from build123d import *

# Parameters (mm, degrees)
BOSS_EXTRUDE1_DEPTH     = 10
CUT_EXTRUDE1_DEPTH      = 44.76694614
CUT_EXTRUDE1_DEPTH_BACK = 44.76694614
SKETCH2_R               = 2.5


with BuildPart() as part:
    # Sketch1 → Boss-Extrude1 (new body)
    with BuildSketch(Plane(origin=(0, 0, 0), x_dir=(0, 1, 0), z_dir=(0, 0, 1))):
        with BuildLine():
            Line((-10.67628561, 39.844440334), (-9.705714191, 36.222218486))
            ThreePointArc((-9.705714191, 36.222218486), (0, 37.5), (9.705714191, 36.222218486))
            Line((9.705714191, 36.222218486), (10.67628561, 39.844440334))
            ThreePointArc((10.67628561, 39.844440334), (0, 41.25), (-10.67628561, 39.844440334))
        make_face()
    extrude(amount=BOSS_EXTRUDE1_DEPTH)

    # Sketch2 → Cut-Extrude1 (cut, two sides: drawn at the far end of the back side and taken through both)
    with BuildSketch(Plane.YZ.offset(-CUT_EXTRUDE1_DEPTH_BACK)):
        with Locations(Location((0, 5, 0), (0, 0, 270))):
            Circle(SKETCH2_R)
    extrude(amount=CUT_EXTRUDE1_DEPTH + CUT_EXTRUDE1_DEPTH_BACK, mode=Mode.SUBTRACT)


solid = part.part
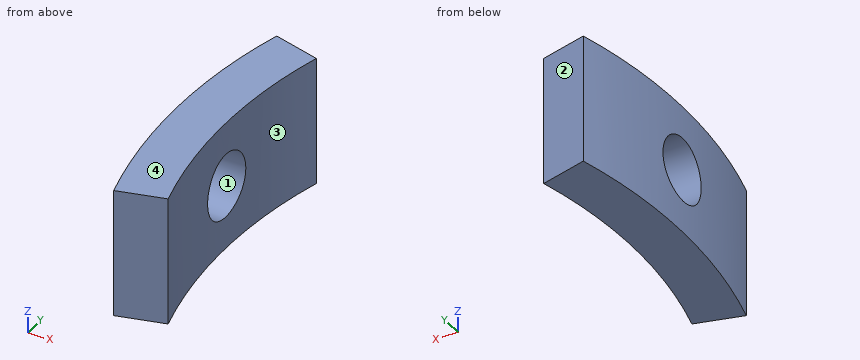
Model file for the job. Use its own axes, mm. Face numbers are marked on the shaded views. Give positions to 0.01 mm unless a question says otherwise; leave off trailing zeros. Order: outer loops, then holes, each group sorted by start corner. A loop starts at its lowest first (then second) coordinate and runs counter-clockwise, first axis right, second up. Notation, with made-up numbers: (89.5, -32) - (115.5, -32) arc R10 ccw to (115.5, -27) - close; hole circle Ø7 at (-30, 68). An arc over 180 degrees is marked (long way). Return JSON: item names as keys, results as strings.
1) Probe line 1 (Z direction, x = -39.3, y = 0); line 2 (Y direction, x = -38.8, z = 5.5); line 3 (Y direction, x = -38.8, z = 5). List the from-to ranges inside material, lowest first. Write a range as from..to.
Geometry says:
{"line 1": "0..2.5, 7.5..10", "line 2": "-10.4..-2.45, 2.45..10.4", "line 3": "-10.4..-2.5, 2.5..10.4"}
2) Cut at C-C, the plane x = -39.35. Give the cut face in (y, z), plus the area to 3 significant figures.
Geometry says:
{"outline": "(-10.54, 0) - (10.54, 0) - (10.54, 10) - (-10.54, 10) - close; hole circle Ø5 at (0, 5)", "area": "191 mm²"}
3) Pull direction Y, two halves, no side cores. Call the marked faces 1, 2, 3 and 4: pulls with the +Y half, pulls with the -Y half, needs draft (parallel to the pull), parting line crosses it, or undercut.
Geometry says:
{"face 1": "undercut", "face 2": "pulls with the +Y half", "face 3": "undercut", "face 4": "needs draft"}
4) Cut at D-D, the plane z = 1.75. Give the cut face in (x, y), plus the area to 3 significant figures.
Geometry says:
{"outline": "(-39.84, -10.68) - (-36.22, -9.71) arc R37.5 cw to (-36.22, 9.71) - (-39.84, 10.68) arc R41.25 ccw to start", "area": "77.3 mm²"}
5) Flat gauge pins, fed straight in: P1, Ø1, axis at y = 5.5, z = 1.5, coming from the -X side; P2, Ø5, axis at y = -7, z = 8.5, coming from the +X side. Where does each tip first touch, or does it go through?
Geometry says:
{"P1": "x = -40.95", "P2": "x = -36.28"}
6) Cut at A-A, the plane y = 0. Give the cut face in (x, z).
Geometry says:
{"outline": "(-41.25, 0) - (-37.5, 0) - (-37.5, 2.5) - (-41.25, 2.5) - close; (-41.25, 7.5) - (-37.5, 7.5) - (-37.5, 10) - (-41.25, 10) - close"}
7) Cut at B-B, the plane z = 6. Give the cut face in (x, y), plus the area to 3 significant figures.
Geometry says:
{"outline": "(-41.19, -2.29) arc R41.25 ccw to (-39.84, -10.68) - (-36.22, -9.71) arc R37.5 cw to (-37.43, -2.29) - close; (-41.19, 2.29) - (-37.43, 2.29) arc R37.5 cw to (-36.22, 9.71) - (-39.84, 10.68) arc R41.25 ccw to start", "area": "60.1 mm²"}
